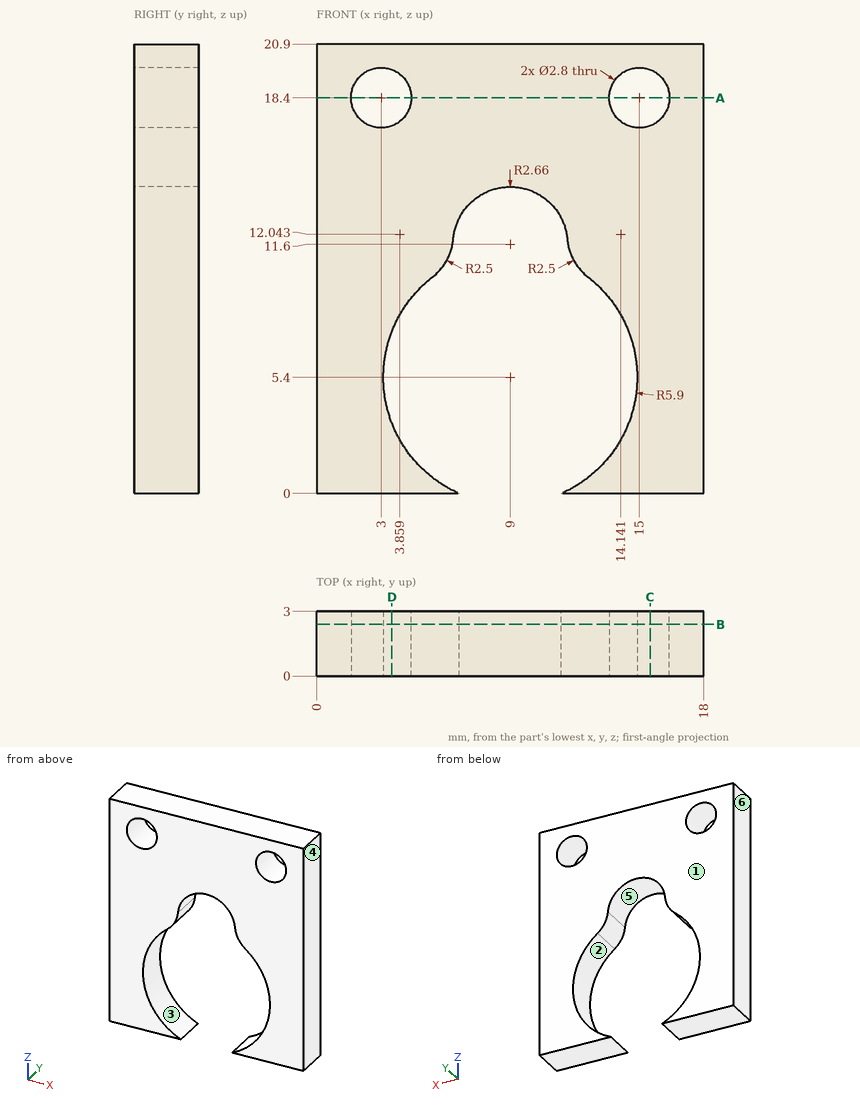
Job drawing, mm, ordinate dimensions from the low corner. One solid piece. A direction names the side the tool comes from. Round coordinates to 2 decimals unless told otherwise and drop trailing zeros. Loops run counter-clockwise (first coordinate to the right, second up) from the corner with the lowest first, then second, coordinate; pieces in that order, holes last. Notation, with made-up numbers: (52, -11.75) -> (90, -11.75) arc R24 ccw to (90, 19.25) -> close; hole circle Ø7 at (-21.5, -32.75). An arc over 180 degrees is marked (long way). Use a Markdown table: item, result.
1) Cut at C-C, the plane x = 15.5. List the corners of the cut face in (y, z).
The answers:
| item | result |
|---|---|
| outline | (0, 0) -> (3, 0) -> (3, 17.09) -> (0, 17.09) -> close; (0, 19.71) -> (3, 19.71) -> (3, 20.9) -> (0, 20.9) -> close |
2) Cut at D-D, the plane x = 3.5. List the corners of the cut face in (y, z) (1 decimal).
The answers:
| item | result |
|---|---|
| outline | (0, 0) -> (3, 0) -> (3, 3.3) -> (0, 3.3) -> close; (0, 7.5) -> (3, 7.5) -> (3, 17.1) -> (0, 17.1) -> close; (0, 19.7) -> (3, 19.7) -> (3, 20.9) -> (0, 20.9) -> close |
3) Tool access for the marked faces 5 and 6: list every direction of +Z, -Z, +X, -X, +Y, -Y with a clear straight run to the whole face (end or side of a thin tool).
The answers:
| item | result |
|---|---|
| face 5 | +Y, -Y |
| face 6 | +Z, -Z, -X, +Y, -Y |
4) Probe line 1 (Z direction, x = 15, y = 0.85); line 2 (Z direction, x = 4, y = 0.45); line 3 (X direction, y = 0.25, z = 5.25). List the from-to ranges inside material, lowest first. Write a range as [from, to].
The answers:
| item | result |
|---|---|
| line 1 | z = [0, 17], [19.8, 20.9] |
| line 2 | z = [0, 2.27], [8.53, 17.42], [19.38, 20.9] |
| line 3 | x = [0, 3.1], [14.9, 18] |
5) Cut at A-A, the plane z = 18.4. List the corners of the cut face in (x, y), and give its area (3 significant figures).
The answers:
| item | result |
|---|---|
| outline | (0, 0) -> (1.6, 0) -> (1.6, 3) -> (0, 3) -> close; (4.4, 0) -> (13.6, 0) -> (13.6, 3) -> (4.4, 3) -> close; (16.4, 0) -> (18, 0) -> (18, 3) -> (16.4, 3) -> close |
| area | 37.2 mm2 |
6) Pull direction X, two halves, no side cores. Call the marked faces 1, 2, 3 and 4: pulls with the +X half, pulls with the -X half, needs draft (parallel to the pull), parting line crosses it, or undercut.
The answers:
| item | result |
|---|---|
| face 1 | needs draft |
| face 2 | undercut |
| face 3 | undercut |
| face 4 | pulls with the +X half |
7) Cut at B-B, the plane y = 2.4. List the corners of the cut face in (x, z), and give its area (3 significant figures).
The answers:
| item | result |
|---|---|
| outline | (0, 0) -> (6.62, 0) arc R5.9 cw to (5.39, 10.07) arc R2.5 ccw to (6.35, 11.83) arc R2.66 cw to (11.65, 11.83) arc R2.5 ccw to (12.61, 10.07) arc R5.9 cw to (11.38, 0) -> (18, 0) -> (18, 20.9) -> (0, 20.9) -> close; hole circle Ø2.8 at (3, 18.4); hole circle Ø2.8 at (15, 18.4) |
| area | 242 mm2 |
